The listing builds one solid part. Answer for the finished solid, in the listing's coordinates (mm). Give positions to 0.01 mm unless a question says otherwise; leave off trailing zeros. Write each loop counter-clockwise with the first axis right and the second up, starting at its lowest first coordinate (ties: lowest second). Pieces come first, ordered by that corner, then holes. Notation, with made-up numbers: M -4.5,20 L 53.5,20 A13 ccw 53.5,37 Z; hole C 73,39.5 d5. An arc over 180 degrees is marked long. Answer as a JSON object with one key per item and string values.
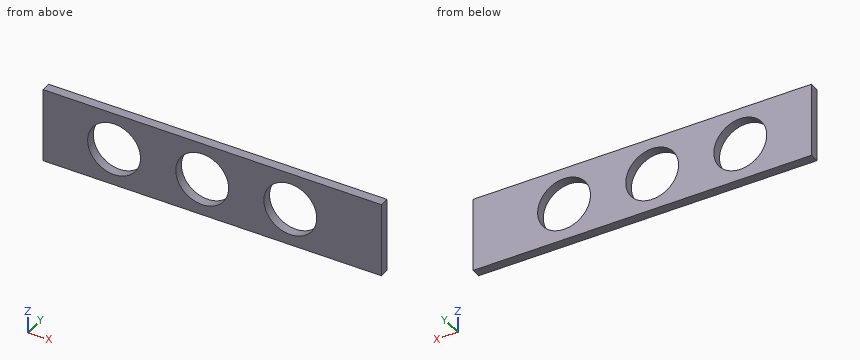
```python
from build123d import *

# Parameters (mm, degrees)
SKETCH_1_W          = 288
SKETCH_1_H          = 63
EXTRUDE_1_DEPTH     = 8
SKETCH_2_R          = 22.5
CUT_EXTRUDE_1_DEPTH = 8
SKETCH_2_3_R        = 22.5
CUT_EXTRUDE_2_DEPTH = 8
SKETCH_2_4_R        = 22.5
CUT_EXTRUDE_3_DEPTH = 8


with BuildPart() as part:
    # Sketch 1 → Extrude 1 (new body)
    with BuildSketch(Plane(origin=(0, 0, 0), x_dir=(1, 0, 0), z_dir=(0, 1, 0))):
        with Locations((144, 31.5)):
            Rectangle(SKETCH_1_W, SKETCH_1_H)
    extrude(amount=EXTRUDE_1_DEPTH)

    # Sketch 2 → Cut-Extrude 1 (cut)
    with BuildSketch(Plane(origin=(0, 8, 0), x_dir=(1, 0, 0), z_dir=(0, 1, 0))):
        with Locations(Location((60.5, 31.5, 0), (0, 0, 270))):
            Circle(SKETCH_2_R)
    extrude(amount=-CUT_EXTRUDE_1_DEPTH, mode=Mode.SUBTRACT)

    # Sketch 2_3 → Cut-Extrude 2 (cut)
    with BuildSketch(Plane(origin=(0, 8, 0), x_dir=(1, 0, 0), z_dir=(0, 1, 0))):
        with Locations(Location((135.5, 31.5, 0), (0, 0, 270))):
            Circle(SKETCH_2_3_R)
    extrude(amount=-CUT_EXTRUDE_2_DEPTH, mode=Mode.SUBTRACT)

    # Sketch 2_4 → Cut-Extrude 3 (cut)
    with BuildSketch(Plane(origin=(0, 8, 0), x_dir=(1, 0, 0), z_dir=(0, 1, 0))):
        with Locations(Location((210.5, 31.5, 0), (0, 0, 270))):
            Circle(SKETCH_2_4_R)
    extrude(amount=-CUT_EXTRUDE_3_DEPTH, mode=Mode.SUBTRACT)


solid = part.part
```
1. A cutting plane is placed at C-C, the plane x = 135.5. Give the vertices of the cut face in (y, z).
Verdict:
{"outline": "M 0,-63 L 8,-63 L 8,-54 L 0,-54 Z; M 0,-9 L 8,-9 L 8,0 L 0,0 Z"}
2. Consider line 1 along X through (y, z) = (2, -33); line 2 along X through (y, z) = (2.75, -31.5); line 3 along Z through (x, y) = (42.5, 0.5). Determine where each line is inside the solid, lowest interval first.
Verdict:
{"line 1": "x = 0 to 38.05, 82.95 to 113.05, 157.95 to 188.05, 232.95 to 288", "line 2": "x = 0 to 38, 83 to 113, 158 to 188, 233 to 288", "line 3": "z = -63 to -45, -18 to 0"}
3. A cutting plane is placed at A-A, the plane y = 6.25. Give the vertices of the cut face in (x, z), plus the area to 3 significant figures.
Verdict:
{"outline": "M 0,-63 L 288,-63 L 288,0 L 0,0 Z; hole C 60.5,-31.5 d45; hole C 135.5,-31.5 d45; hole C 210.5,-31.5 d45", "area": "13,400 mm2"}
4. A cutting plane is placed at D-D, the plane x = 75.5. Give the vertices of the cut face in (y, z).
Verdict:
{"outline": "M 0,-63 L 8,-63 L 8,-48.27 L 0,-48.27 Z; M 0,-14.73 L 8,-14.73 L 8,0 L 0,0 Z"}
5. A cutting plane is placed at B-B, the plane z = -31.5. Give the vertices of the cut face in (x, y).
Verdict:
{"outline": "M 0,0 L 38,0 L 38,8 L 0,8 Z; M 83,0 L 113,0 L 113,8 L 83,8 Z; M 158,0 L 188,0 L 188,8 L 158,8 Z; M 233,0 L 288,0 L 288,8 L 233,8 Z"}
